Model file for the job. Use its own axes, mm. Face numbers are marked on the shaded views. A direction names the side the tool comes from. Coordinates: 2 decimals unless noted, no trailing zeros. Put each result on its own line as item: value. Start each with the question number.
```python
from build123d import *

# Parameters (mm, degrees)
BOSS_EXTRUDE1_DEPTH     = 16.668
CUT_EXTRUDE1_DEPTH      = 45.45
CUT_EXTRUDE1_DEPTH_BACK = 45.45
DRAFT1_ANGLE            = 1
CUT_EXTRUDE2_REACH      = 38.469
SKETCH3_R               = 5.5
CUT_EXTRUDE4_REACH      = 38.469
SKETCH5_R               = 5.5
FILLET1_R               = 3


with BuildPart() as part:
    # Sketch1 → Boss-Extrude1 (new body, symmetric)
    with BuildSketch(Plane(origin=(0, 0, 0), x_dir=(0, 0, -1), z_dir=(1, 0, 0))):
        with BuildLine():
            Line((22.225, 38.494829198), (45.45, 25.085869196))
            Line((45.45, 25.085869196), (45.45, -25.085869196))
            Line((45.45, -25.085869196), (22.225, -38.494829198))
            ThreePointArc((22.225, -38.494829198), (-44.45, 0), (22.225, 38.494829198))
        make_face()
    extrude(amount=BOSS_EXTRUDE1_DEPTH, both=True)

    # Sketch2 → Cut-Extrude1 (cut, two sides)
    with BuildSketch(Plane(origin=(0, 0, 0), x_dir=(1, 0, 0), z_dir=(0, 1, 0))) as cut_extrude1_sk:
        with BuildLine():
            Line((-7.588316422, 21.130183578), (-0.129046134, 13.670913289))
            Line((-0.129046134, 13.670913289), (-1.143550449, -44.45))
            Line((-1.143550449, -44.45), (1.143550449, -44.45))
            Line((1.143550449, -44.45), (0.129046134, 13.670913289))
            Line((0.129046134, 13.670913289), (7.588316422, 21.130183578))
            ThreePointArc((7.588316422, 21.130183578), (0, 39.45), (-7.588316422, 21.130183578))
        make_face()
    extrude(amount=CUT_EXTRUDE1_DEPTH, mode=Mode.SUBTRACT)
    extrude(cut_extrude1_sk.sketch, amount=-CUT_EXTRUDE1_DEPTH_BACK, mode=Mode.SUBTRACT)

    # Draft1
    draft1_faces = [part.faces().sort_by_distance(p)[0] for p in [
        (16.668, 0, -1.658648034),
        (-16.668, 0, -1.658648034),
    ]]
    draft(draft1_faces, Plane(origin=(16.668, 25.085869196, -45.45), x_dir=(-1, 0, 0), z_dir=(0, 0, -1)), DRAFT1_ANGLE)

    # Sketch3 → Cut-Extrude2 (cut, up to next)
    with BuildSketch(Plane(origin=(17.456014215, 0, -0.304695862), x_dir=(-0.017452406, 0, -0.999847695), z_dir=(0.999847695, 0, -0.017452406)), mode=Mode.PRIVATE) as cut_extrude2_sk1:
        with Locations((-0.304742275, 0)):
            Circle(SKETCH3_R)
    cut_extrude2_tool1 = extrude(cut_extrude2_sk1.sketch, amount=-CUT_EXTRUDE2_REACH, mode=Mode.PRIVATE) & part.part
    add(cut_extrude2_tool1.solids().sort_by_distance((17.461333, 0, 0))[0], mode=Mode.SUBTRACT)

    # Sketch5 → Cut-Extrude4 (cut, up to next)
    with BuildSketch(Plane(origin=(-17.456014215, 0, -0.304695862), x_dir=(-0.017452406, 0, 0.999847695), z_dir=(-0.999847695, 0, -0.017452406)), mode=Mode.PRIVATE) as cut_extrude4_sk1:
        with Locations((0.304742275, 0)):
            Circle(SKETCH5_R)
    cut_extrude4_tool1 = extrude(cut_extrude4_sk1.sketch, amount=-CUT_EXTRUDE4_REACH, mode=Mode.PRIVATE) & part.part
    add(cut_extrude4_tool1.solids().sort_by_distance((-17.461333, 0, 0))[0], mode=Mode.SUBTRACT)

    # Fillet1
    fillet1_edges = [part.edges().sort_by_distance(p)[0] for p in [
        (16.870696941, 31.790349197, -33.8375),
        (18.237210337, 0.000220739, 44.449999999),
        (-16.870696941, 31.790349197, -33.8375),
        (-16.870697084, -31.790353899, -33.837491856),
        (-18.237210337, 9.404e-06, 44.45),
        (16.870700278, -31.790459554, -33.837308856),
    ]]
    fillet(fillet1_edges, radius=FILLET1_R)


solid = part.part
```
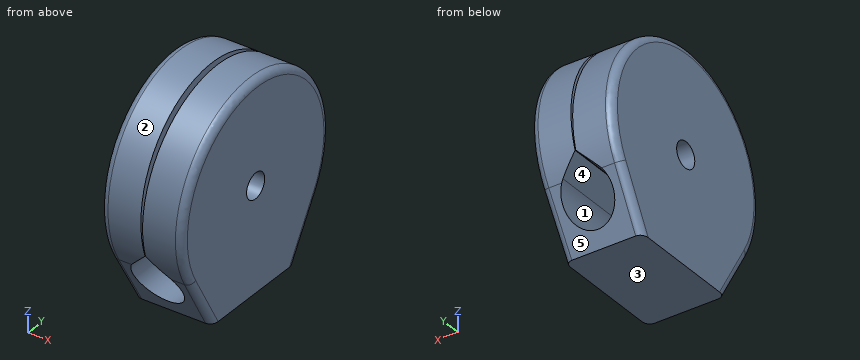
Item 1: Flat gauge pins, fed straight in: pin 1 Ø4 at (x, z) = (-11, 26.5) entering from +Y; pin 2 Ø2 at (x, z) = (-3, 14.5) entering from -Y; pin 3 Ø8 at (y, z) = (31.5, 5.5) entering from +X; pin 4 Ø13 at (x, z) = (0, -28.72) entering from -Y. Where does each tip first touch, or does it go through?
Item 2: Pull direction Z, two halves, no side cores. Call the marked faces 1, 2 and 3: pulls with the +Z half, pulls with the -Z half, needs draft (parallel to the pull), parting line crosses it, or undercut.
Item 3: 3-axis set-ups, long thin cutter, end or side, ignore diameter. For the marked faces 4 and 5: which of +Z, -Z, +X, -X, +Y, -Y reach the whole face in a straight line?
Item 4: Slice it at A-A, the plane x = 3. Give the number of separate pieces and of enclosed holes in the cut face, plus the area to 3 significant figures.
Item 5: Wall check: line 1 along Z through (x, y) = (-7.5, -3); line 2 along Z through (x, y) = (-9, 0.5); line 3 along Z through (x, y) = (0, 23.5). Give the ranges that are in metal, low to high.
Here are the results:
1. pin 1: stops at y = 37.09
1. pin 2: stops at y = -42.35
1. pin 3: stops at x = 17.63
1. pin 4: passes through
2. face 1: undercut
2. face 2: parting line crosses it
2. face 3: pulls with the -Z half
3. face 4: +Y, -Y
3. face 5: -Z, +X, -X, +Y
4. separate pieces: 2
4. enclosed holes: 1
4. area: 4,790 mm^2
5. line 1: z = -45.45 to -36.39, -21.04 to -4.44, 4.78 to 44.35
5. line 2: z = -45.45 to -34.56, -22.87 to -5.33, 5.63 to 44.45
5. line 3: z = -45.45 to -39.45
